from build123d import *

# Parameters (mm, degrees)
BOSS_EXTRUDE1_DEPTH   = 5.9944
SKETCH2_R             = 5.08
CUT_EXTRUDE1_DEPTH    = 381.139257342
CUT_EXTRUDE2_DEPTH    = 1.27
FILLET1_R             = 6.35
BODY_MOVE_COPY1_ANGLE = 90


with BuildPart() as part:
    # Sketch1 → Boss-Extrude1 (new body)
    with BuildSketch(Plane(origin=(0, 0, 0), x_dir=(1, 0, 0), z_dir=(0, 1, 0))):
        Polygon((-63.5, 0), (63.5, 0), (134.23323784, -355.6), (-134.23323784, -355.6), align=None)
    extrude(amount=BOSS_EXTRUDE1_DEPTH)

    # Sketch2 → Cut-Extrude1 (cut, through all)
    with BuildSketch(Plane(origin=(0, 5.9944, 0), x_dir=(1, 0, 0), z_dir=(0, 1, 0))):
        with Locations(Location((0, -101.6, 0), (0, 0, 270))):
            Circle(SKETCH2_R)
    extrude(amount=-CUT_EXTRUDE1_DEPTH, mode=Mode.SUBTRACT)

    # Sketch3 → Cut-Extrude2 (cut)
    # profile 1 of 2: a face of its own
    with BuildSketch(Plane(origin=(0, 5.9944, 0), x_dir=(1, 0, 0), z_dir=(0, 1, 0))):
        Polygon((-5.958315024, -115.820937251), (-4.079773357, -115.820937251), (-4.079773357, -125.980937251), (-4.991568229, -125.980937251), (-4.991568229, -116.862988533), (-6.554645152, -116.862988533), align=None)
    # profile 2 of 2: a face of its own
    with BuildSketch(Plane(origin=(0, 5.9944, 0), x_dir=(1, 0, 0), z_dir=(0, 1, 0))):
        with BuildLine():
            Line((4.386893309, -115.56042443), (5.089056771, -116.111978917))
            Line((5.089056771, -116.111978917), (2.404553566, -120.217091097))
            add(Edge.make_bspline(
                [(2.404553566, -120.217091097), (2.583283284, -120.188602861), (2.931915808, -120.133033337), (3.284804245, -120.123866273), (3.45678113, -120.119398789)],
                knots=[0, 0, 0, 0, 1.025318673, 2, 2, 2, 2], degree=3))
            add(Edge.make_bspline(
                [(3.45678113, -120.119398789), (3.560043005, -120.122174245), (3.763310933, -120.127637647), (4.061744393, -120.169682196), (4.348514562, -120.235940235), (4.622432842, -120.332524841), (4.884482412, -120.455903104), (5.136167082, -120.603771368), (5.372755774, -120.783765), (5.597295197, -120.984831271), (5.801154428, -121.207529718), (5.981642635, -121.44382617), (6.133249551, -121.693474441), (6.256254992, -121.956348086), (6.351773154, -122.232041891), (6.42140586, -122.520203119), (6.462567193, -122.821030476), (6.468156617, -123.025618551), (6.470995873, -123.12954302)],
                knots=[0, 0, 0, 0, 1.04369286, 2.054478336, 3.041073146, 4.015093852, 4.984733326, 5.965804835, 6.960378782, 7.985147595, 9.009457201, 10.008161701, 10.986880575, 11.956520048, 12.937015923, 13.931873656, 14.949455224, 16, 16, 16, 16], degree=3))
            add(Edge.make_bspline(
                [(6.470995873, -123.12954302), (6.466864803, -123.271724103), (6.458735835, -123.551502827), (6.377735101, -123.958996352), (6.251868247, -124.34720274), (6.071956336, -124.709923946), (5.848487475, -125.046662834), (5.575974235, -125.345034357), (5.264081137, -125.611139379), (4.911422318, -125.833662594), (4.53189417, -126.015390308), (4.133180944, -126.145917982), (3.719154713, -126.226279139), (3.438144765, -126.236353802), (3.295995873, -126.241450071)],
                knots=[0, 0, 0, 0, 1.031375318, 2.029502543, 3.004789286, 3.987476834, 4.960371455, 5.9300674, 6.912260825, 7.929083631, 8.949397511, 9.960523116, 10.96833055, 12, 12, 12, 12], degree=3))
            add(Edge.make_bspline(
                [(3.295995873, -126.241450071), (3.15928088, -126.237013908), (2.888472414, -126.228226646), (2.490105217, -126.149948381), (2.107325715, -126.023072905), (1.742815741, -125.848279457), (1.405153618, -125.627494288), (1.103065942, -125.361702072), (0.838058963, -125.056584311), (0.617515491, -124.712188331), (0.442593001, -124.342103197), (0.311413104, -123.956205623), (0.234788581, -123.555901676), (0.224081227, -123.284539284), (0.218688181, -123.147860328)],
                knots=[0, 0, 0, 0, 1.012016664, 2.004627821, 2.994792927, 3.992885782, 4.990978636, 5.973936114, 6.964471063, 7.975201453, 8.993600317, 9.990122807, 10.98767138, 12, 12, 12, 12], degree=3))
            add(Edge.make_bspline(
                [(0.218688181, -123.147860328), (0.222117747, -123.043228052), (0.229120266, -122.829588936), (0.278014222, -122.506024787), (0.356579455, -122.174950789), (0.44456577, -121.894087187), (0.537531541, -121.664002312), (0.614900056, -121.478499608), (0.711199427, -121.287604607), (0.813883299, -121.084771424), (0.932194667, -120.875227425), (1.060836667, -120.655470487), (1.203365939, -120.428995588), (1.303282754, -120.275306153), (1.354361258, -120.196738533)],
                knots=[0, 0, 0, 0, 1.173818275, 2.396712641, 3.66331629, 4.989737886, 5.693666774, 6.447286557, 7.243889047, 8.091586357, 8.998013824, 9.943181721, 10.948533338, 12, 12, 12, 12], degree=3))
            Line((1.354361258, -120.196738533), (4.386893309, -115.56042443))
        make_face()
        with BuildLine():
            add(Edge.make_bspline(
                [(3.265467027, -121.161450071), (3.188070339, -121.163708621), (3.036892125, -121.168120225), (2.815092315, -121.19373867), (2.605177277, -121.241981443), (2.40436594, -121.303424281), (2.216412608, -121.387906306), (2.03995129, -121.490527528), (1.874299597, -121.611347862), (1.721192601, -121.74865565), (1.58237895, -121.898988912), (1.46283601, -122.06000901), (1.359719557, -122.227835383), (1.275879763, -122.403870278), (1.210594286, -122.588046402), (1.163369878, -122.77951668), (1.137088131, -122.979565066), (1.132715756, -123.115222846), (1.130483053, -123.184494943)],
                knots=[0, 0, 0, 0, 1.129588631, 2.206414736, 3.251139165, 4.268635594, 5.265702196, 6.250456724, 7.242448911, 8.251968645, 9.246821453, 10.222880186, 11.173611482, 12.116736599, 13.062300278, 14.020270554, 14.989073742, 16, 16, 16, 16], degree=3))
            add(Edge.make_bspline(
                [(1.130483053, -123.184494943), (1.132301291, -123.253147456), (1.135866585, -123.387764814), (1.168240176, -123.586143689), (1.217690586, -123.777049823), (1.291250136, -123.959499036), (1.378994474, -124.136272348), (1.494833929, -124.300966776), (1.623188942, -124.463585037), (1.77661636, -124.611635023), (1.941276179, -124.749394823), (2.117192813, -124.869806073), (2.300537154, -124.972817365), (2.493784482, -125.053549009), (2.694193048, -125.119804653), (2.903432599, -125.166428832), (3.121648659, -125.192788302), (3.269467771, -125.197166373), (3.344842027, -125.199398789)],
                knots=[0, 0, 0, 0, 0.989467248, 1.94019797, 2.891935182, 3.827694429, 4.772920941, 5.730924762, 6.725747692, 7.756678648, 8.79901574, 9.819492441, 10.826891316, 11.826466727, 12.835195252, 13.867842842, 14.912794438, 16, 16, 16, 16], degree=3))
            add(Edge.make_bspline(
                [(3.344842027, -125.199398789), (3.42021616, -125.197166198), (3.568035029, -125.192787784), (3.786252845, -125.166430802), (3.995485908, -125.119797424), (4.195918058, -125.053575211), (4.389078327, -124.972720162), (4.572262318, -124.870446932), (4.746515298, -124.748654316), (4.91128321, -124.611870444), (5.064072014, -124.462742394), (5.195505486, -124.3024184), (5.307797386, -124.134941263), (5.399046341, -123.960195389), (5.471795689, -123.776939505), (5.521496863, -123.586173243), (5.553803599, -123.387757076), (5.557378079, -123.253144843), (5.559201002, -123.184494943)],
                knots=[0, 0, 0, 0, 1.087397944, 2.132534446, 3.165364764, 4.174271784, 5.174024072, 6.181601208, 7.194203697, 8.236725232, 9.267838612, 10.269026844, 11.221737037, 12.171628256, 13.107553087, 14.05945871, 15.010357665, 16, 16, 16, 16], degree=3))
            add(Edge.make_bspline(
                [(5.559201002, -123.184494943), (5.55760358, -123.115132475), (5.55446836, -122.978996509), (5.519007206, -122.779606166), (5.469825915, -122.587073567), (5.395562032, -122.402608755), (5.299081091, -122.226939663), (5.181563543, -122.059178902), (5.045615282, -121.898040294), (4.888577853, -121.748360827), (4.717627917, -121.611499595), (4.535863817, -121.490683969), (4.345703528, -121.388721179), (4.147339855, -121.303646848), (3.938499944, -121.242252946), (3.722555417, -121.19391096), (3.496744358, -121.168185789), (3.343541404, -121.163723908), (3.265467027, -121.161450071)],
                knots=[0, 0, 0, 0, 0.978206639, 1.919901502, 2.851605144, 3.780102724, 4.718870031, 5.675451981, 6.667674623, 7.690630536, 8.733308323, 9.756129687, 10.767539656, 11.776269907, 12.797430371, 13.836405707, 14.897401972, 16, 16, 16, 16], degree=3))
        make_face(mode=Mode.SUBTRACT)
    extrude(amount=-CUT_EXTRUDE2_DEPTH, mode=Mode.SUBTRACT)

    # Fillet1
    fillet1_edges = [part.edges().sort_by_distance(p)[0] for p in [
        (134.23323784, 2.9972, 355.6),
        (-134.23323784, 2.9972, 355.6),
        (-63.5, 2.9972, 0),
        (63.5, 2.9972, 0),
    ]]
    fillet(fillet1_edges, radius=FILLET1_R)


with BuildPart() as part_1:
    # Body-Move/Copy1: moved
    add(part.part.rotate(Axis((0, 0, 177.8), (0, 1, 0)), BODY_MOVE_COPY1_ANGLE))


solid = part_1.part
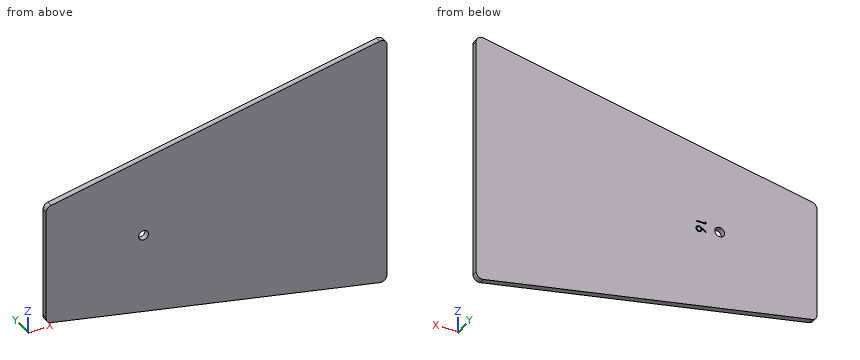
Build history of the part. All positions in model axes, mm. Coordinates: 2 decimals unless noted, no trailing zeros. Write each loop counter-clockwise with the first axis right and the second up, starting at its lowest first coordinate (ties: lowest second). Pieces come first, ordered by that corner, then holes.
(1) Cut at B-B on x = -76.2. List the corners of the cut face in (y, z), and give its area (3 significant figures).
(2) Drill centre lines: line 1 (X direction, y = 1.5, z = 177.8); line 2 (Z direction, x = -76.2, y = 4.1); line 3 (Z direction, x = -139, y = 3.9). Where is each one in solid material? Low to high.
(3) Cut at C-C on z = 262. List the corners of the cut face in (x, y).
(4) Pin check, flat tips, straight feed: pin 1 Ø1 at (x, y) = (-55.5, 5) entering from +Z; pin 2 Ø1.4 at (x, y) = (-56.5, 5.5) entering from -Z; pin 3 Ø2 at (x, y) = (-103.5, 5) entering from +Z. Stop position of each tip, or through.
(5) Cut at A-A on y = 3.6. List the corners of the cut face in (x, z), and give its area (3 significant figures).
(6) Cut at D-D on x = 64. List the corners of the cut face in (y, z).
Working result:
1. outline: (0, 94.09) - (5.99, 94.09) - (5.99, 172.72) - (0, 172.72) - close; (0, 182.88) - (5.99, 182.88) - (5.99, 261.51) - (0, 261.51) - close
1. area: 943 mm2
2. line 1: x = -177.8 to -81.28, -71.12 to 177.8
2. line 2: z = 94.09 to 172.72, 182.88 to 261.51
2. line 3: z = 106.58 to 249.02
3. outline: (-73.73, 0) - (177.8, 0) - (177.8, 5.99) - (-73.73, 5.99) - close
4. pin 1: stops at z = 265.73
4. pin 2: stops at z = 90.03
4. pin 3: stops at z = 256.28
5. outline: (-177.8, 119.51) arc R6.35 ccw to (-172.69, 113.28) - (170.21, 45.08) arc R6.35 ccw to (177.8, 51.3) - (177.8, 304.3) arc R6.35 ccw to (170.21, 310.52) - (-172.69, 242.32) arc R6.35 ccw to (-177.8, 236.09) - close; hole circle Ø10.16 at (-76.2, 177.8)
5. area: 70,200 mm2
6. outline: (0, 66.2) - (5.99, 66.2) - (5.99, 289.4) - (0, 289.4) - close
